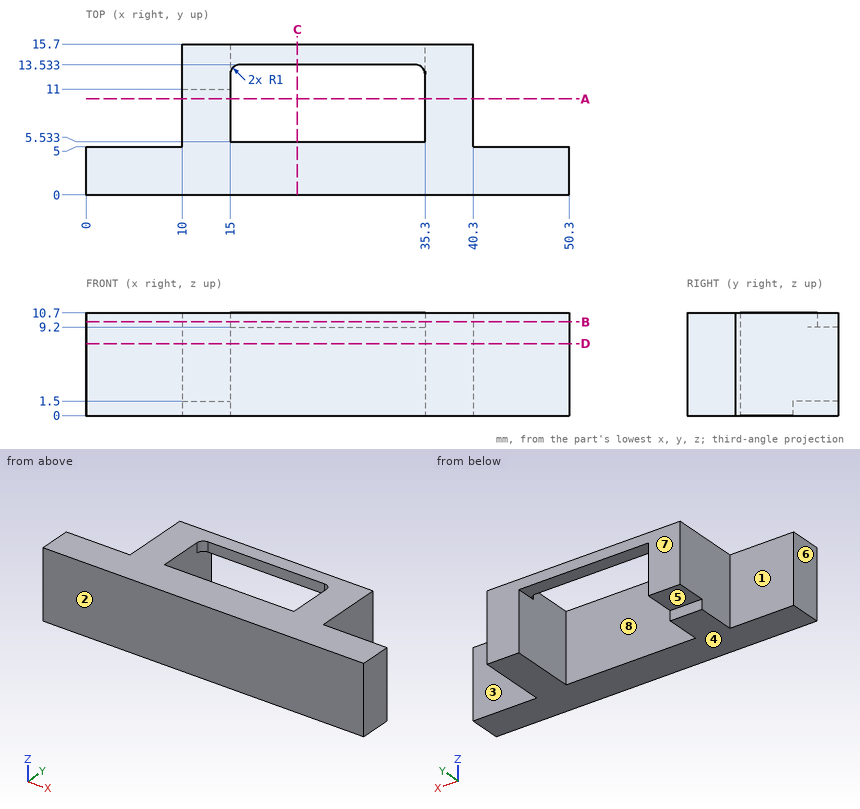
Here's the drawing with two shaded views (mm, measured from the low corner). I have some questions. A direction names the side the tool comes from. Coordinates: 2 decimals unless noted, no trailing zeros. Loops run counter-clockwise (first coordinate to the right, second up) from the corner with the lowest first, then second, coordinate; pieces in that order, holes last. Notation, with made-up numbers: (77, 59.5) -> (102, 59.5) arc R27 cw to (102, 80.5) -> close; hole circle Ø5 at (-28, 19.25). An arc over 180 degrees is marked (long way). Use one line per item in the form item = value. Start each with the question number.
(1) If we section it at D-D (z = 7.5): Please give me the cut outline in (x, y), then the cut area to 3 significant figures.
(2) On a 3-axis mill with a long thin cutter (end or side, diameter ignored), from which of +Z, -Z, +X, -X, +Y, -Y can I reach the whole of each face in a straight line? I mean the marked faces 1, 2, 3, 4 and 5. Say none if no direction works.
(3) If we section it at A-A (y = 10): Please give me the cut outline in (x, z), then the cut area to 3 significant figures.
(4) Please list where these lines run through material, in increasing order: line 1 along X through (y, z) = (11.25, 6.5); line 2 along Y through (x, z) = (16, 10); line 3 along Y through (x, z) = (16, 8).
(5) If we section it at C-C (x = 22): Please give me the cut outline in (y, z).
(6) If we section it at B-B (z = 9.75): Please give me the cut outline in (x, y).
(7) Will these pins go through, and if not, where does the flat tip stop? pin 1 (6 mm diameter, centred on x = 22, y = 12.5, fed in from -Z); pin 2 (1.5 mm diameter, centred on x = 34, y = 7, fed in from +Z); pin 3 (5 mm diameter, centred on x = 43.5, z = 3.5, fed in from +Y); pin 4 (3 mm diameter, centred on y = 8.5, z = 3, fed in from -X).
(8) We'd pull the mould along X, two halves only. Please class the marked faces 6, 7 and 8: pulls with the +X half, pulls with the -X half, needs draft (parallel to the pull), parting line crosses it, or undercut.
Verdict:
q1.outline = (0, 0) -> (50.3, 0) -> (50.3, 5) -> (40.3, 5) -> (40.3, 15.7) -> (35.3, 15.7) -> (35.3, 5.53) -> (15, 5.53) -> (15, 15.7) -> (10, 15.7) -> (10, 5) -> (0, 5) -> close
q1.area = 369 mm²
q2.face_1 = +Z, -Z, -X, +Y
q2.face_2 = +Z, -Z, +X, -X, -Y
q2.face_3 = +Z, -Z, +X, +Y
q2.face_4 = -Z, +X, -X, +Y, -Y
q2.face_5 = -Z, -X, +Y
q3.outline = (10, 0) -> (15, 0) -> (15, 10.7) -> (10, 10.7) -> close; (35.3, 0) -> (40.3, 0) -> (40.3, 10.7) -> (35.3, 10.7) -> close
q3.area = 107 mm²
q4.line_1 = 10 to 15, 35.3 to 40.3
q4.line_2 = 0 to 5.53, 13.53 to 15.7
q4.line_3 = 0 to 5.53
q5.outline = (0, 0) -> (5.53, 0) -> (5.53, 10.7) -> (0, 10.7) -> close; (13.53, 9.2) -> (15.7, 9.2) -> (15.7, 10.7) -> (13.53, 10.7) -> close
q6.outline = (0, 0) -> (50.3, 0) -> (50.3, 5) -> (40.3, 5) -> (40.3, 15.7) -> (10, 15.7) -> (10, 5) -> (0, 5) -> close; hole (15, 5.53) -> (35.3, 5.53) -> (35.3, 12.53) arc R1 ccw to (34.3, 13.53) -> (16, 13.53) arc R1 ccw to (15, 12.53) -> close
q7.pin_1 = 9.2
q7.pin_2 = through
q7.pin_3 = 5
q7.pin_4 = 10
q8.face_6 = pulls with the -X half
q8.face_7 = needs draft
q8.face_8 = undercut
